Can you work these out from the model? Positions are in its coordinate system, mm. A direction names the side the tool comes from. Round coordinates to 2 decimals unless told otherwise and drop trailing zeros. Order: outer loops, then holes, each group sorted by start corner. A loop starts at its lowest first (then second) coordinate and runs counter-clockwise, first axis right, second up. Notation, with made-up numbers: M 41,87 L 98,87 A27 cw 98,121 Z; hole C 43,15.5 d10. An arc over 180 degrees is marked long. Answer as a JSON object with one key per item and string values. Group by question number.
from build123d import *

# Parameters (mm, degrees)
F1_DEPTH = 50
F3_DEPTH = 10
F5_DEPTH = 10
F7_DEPTH = 25.9997663884
F8_R     = 5
F9_R     = 5


with BuildPart() as f1:
    # F0 (on Front) → F1 (new body)
    with BuildSketch(Plane.XZ):
        with BuildLine():
            Line((0, 10), (0, 0))
            Line((0, 0), (30, 0))
            ThreePointArc((30.0000000018, 0), (45.0002337116, 14.9997662866), (59.9999999982, -0.0004674232))
            Line((60, -0.0004674232), (89.9999999964, 0))
            Line((89.9999999964, 0), (89.999610477, 24.999999997))
            Line((89.999610477, 24.999999997), (79.9996104782, 24.9998441892))
            Line((79.9996104782, 24.9998441892), (79.9998441898, 9.999844191))
            Line((79.9998441898, 9.999844191), (67.9129266661, 9.9996558675))
            ThreePointArc((67.9129266661, 9.9996558675), (45.0001877399, 24.9997662877), (22.0872235267, 10))
            Line((22.0872235267, 10), (0, 10))
        make_face()
    extrude(amount=-F1_DEPTH)

    # F2 (on face) → F3 (cut, through all)
    with BuildSketch(Plane(origin=(89.9999999745, 0, 0.0014022697), x_dir=(0, 1, 0), z_dir=(0.9999999999, 0, 1.55808e-05))):
        with BuildLine():
            Line((30, 24.9985977303), (20, 24.9985977303))
            Line((20, 24.9985977303), (20, 14.9985977303))
            ThreePointArc((20, 14.9985977303), (25, 9.9985977303), (30, 14.9985977303))
            Line((30, 14.9985977303), (30, 24.9985977303))
        make_face()
    extrude(amount=-F3_DEPTH, mode=Mode.SUBTRACT)

    # F4 (on face) → F5 (cut, through all)
    with BuildSketch(Plane.XY.offset(10)):
        with BuildLine():
            ThreePointArc((12.0710678119, 42.9289321881), (8.9844849737, 47.5483298507), (3.5355339059, 46.4644660941))
            ThreePointArc((3.5355339059, 46.4644660941), (5.15765065, 38.3095345256), (12.0710678119, 42.9289321881))
        make_face()
        with BuildLine():
            ThreePointArc((12.0710678119, 7.0710678119), (5.15765065, 11.6904654744), (3.5355339059, 3.5355339059))
            ThreePointArc((3.5355339059, 3.5355339059), (8.9844849737, 2.4516701493), (12.0710678119, 7.0710678119))
        make_face()
    extrude(amount=-F5_DEPTH, mode=Mode.SUBTRACT)

    # F6 (on Top) → F7 (cut, up to face)
    with BuildSketch(Plane.XY):
        with BuildLine():
            ThreePointArc((45, 20), (48.5355339059, 21.4644660941), (50, 25))
            ThreePointArc((50, 25), (41.4644660941, 28.5355339059), (45, 20))
        make_face()
    extrude(amount=F7_DEPTH, mode=Mode.SUBTRACT)

    # F8
    f8_edges = [f1.edges().sort_by_distance(p)[0] for p in [
        (0, 0, 5),
        (0, 50, 5),
    ]]
    fillet(f8_edges, radius=F8_R)

    # F9
    f9_edges = [f1.edges().sort_by_distance(p)[0] for p in [
        (84.99961, 0, 24.999922),
        (84.99961, 50, 24.999922),
    ]]
    fillet(f9_edges, radius=F9_R)


solid = f1.part
Item 1: On a 3-axis mill with a long thin cutter (end or side, diameter ignored), from which of +Z, -Z, +X, -X, +Y, -Y can I reach the whole of each face in a straight line? I mean faces 4 (the face through (46.9, 0, 15.5)), 5 (the face through (85, 30, 20)). Say none if no direction works.
Item 2: Suppose I cut it at B-B, the plane y = 35. Write out the boundary of the cut face in (x, z), and give its area (3 significant figures).
Item 3: Suppose I cut it at D-D, the plane x = 27. Write out the boundary of the cut face in (y, z), and give its area (3 significant figures).
Item 4: If we mould it in two halves opening along X, with no side actions, what happens to faces 1 (the face through (11, 25, 10)), 2 (the face through (1, 48, 5)), 3 (the face through (39.56, 24.65, 13.98))? For each: +X half, -X half, draft (parallel to the pull), parting line (faces both ways), or undercut.
Item 5: Suppose I cut it at A-A, the plane z = 5. Write out the boundary of the cut face in (x, y).
Item 6: Suppose I cut it at C-C, the plane z = 23.25. State how many separate pieces and enclosed holes the cut face has, and give its area (3 significant figures).
Item 7: I'm going to push flat-ended pins straight in: pin 1 Ø7.5 at (y, z) = (11, 16) entering from -X; pin 2 Ø1 at (y, z) = (26, 11) entering from -X; pin 3 Ø6 at (x, y) = (38, 18.5) entering from -Z. Where does each tip first touch, or does it pass through?
Item 8: I need wall thicknesses on line 1 (Y direction, x = 4.5, z = 8.5); line 2 (X direction, y = 8.5, z = 22.25); line 3 (X direction, y = 40.5, z = 3.75). Which ranges of each line are inside material? Lowest first, please.
Computed:
{
 "1": {"face 4": "+Z, -Z, +X, -X, -Y", "face 5": "+Z, +X"},
 "2": {"outline": "M 0,0 L 30,0 A15 cw 60,0 L 90,0 L 90,25 L 80,25 L 80,10 L 67.91,10 A25 ccw 22.09,10 L 0,10 Z", "area": "1,190 mm^2"},
 "3": {"outline": "M 0,0 L 50,0 L 50,17.35 L 0,17.35 Z", "area": "867 mm^2"},
 "4": {"face 1": "draft", "face 2": "-X half", "face 3": "undercut"},
 "5": {"outline": "M 0,5 A5 ccw 5,0 L 30.86,0 L 30.86,50 L 5,50 A5 ccw 0,45 Z; M 59.14,0 L 90,0 L 90,50 L 59.14,50 Z; hole C 7.07,7.07 d10; hole C 7.07,42.93 d10"},
 "6": {"separate pieces": "3", "enclosed holes": "1", "area": "1,220 mm^2"},
 "7": {"pin 1": "stops at x = 23.21", "pin 2": "stops at x = 22.31", "pin 3": "stops at z = 11.18"},
 "8": {"line 1": "y = 0.03 to 2.78, 11.36 to 38.64, 47.22 to 49.97", "line 2": "x = 33.6 to 56.4, 80 to 90", "line 3": "x = 0 to 2.7, 11.44 to 30.48, 59.52 to 90"}
}
